Could you check a few things on this model? Use its own coordinates, in mm. A direction names the side the tool comes from. Coordinates: 2 decimals unless noted, no trailing zeros. Order: outer loops, then holes, each group sorted by start corner. A loop starts at its lowest first (then second) coordinate and runs counter-clockwise, first axis right, second up. Notation, with made-up numbers: (-7.75, -33) - (40.25, -33) arc R23 ccw to (40.25, -18) - close; hole circle Ø6 at (-7.75, 51). An arc over 180 degrees is marked (long way). Answer as a JSON object with one key per item and string values. Group by question number.
(1) Which directions (+Z, -Z, +X, -X, +Y, -Y) give clear straight access to the entire face, cutting with the end or side of a thin tool? Please do faces 1 (the flat face through (29.163, 14, 6)), 2 (the flat face through (9, 26, 1)), 3 (the flat face through (20, 58, 4)).
(2) Imagine slicing it at B-B, the plane x = 31. Write out the boundary of the cut face in (y, z), and give its area (3 significant figures).
(3) We'd pull the mould along X, two halves only. Please class faces 4 (the flat face through (20, 28, 3)), 5 (the flat face through (20, 0, 4)): pulls with the +X half, pulls with the -X half, needs draft (parallel to the pull), parting line crosses it, or undercut.
(4) Will these pins go through, and if not, where does the flat tip stop? P1, Ø1.2, axis at x = 28, y = 16, coming from the +Z side; P2, Ø0.9, axis at x = 23, y = 21.5, coming from the -Z side; P3, Ø2, axis at x = 18.5, y = 19, coming from the +Z side.
(5) Imagine slicing it at A-A, the plane y = 33. Write out the boundary of the cut face in (x, z), and give its area (3 significant figures).
(6) Please list where these lines run through material, in increasing order: probe 1 along Y at (x, z) = (5, 2); probe 2 along X at (y, z) = (18.5, 5.75); probe 3 along X at (y, z) = (46.5, 6.5).
(7) Imagine slicing it at C-C, the plane y = 4.5. Write out the boundary of the cut face in (x, z), and give its area (3 significant figures).
(8) Imagine slicing it at D-D, the plane z = 2.75. Write out the boundary of the cut face in (x, y).
from build123d import *

# Parameters (mm, degrees)
SKETCH1_W           = 60
SKETCH1_H           = 40
BOSS_EXTRUDE1_DEPTH = 8
SKETCH3_R           = 1.15
CUT_EXTRUDE2_DEPTH  = 73.553428589
SKETCH7_W           = 25
SKETCH7_H           = 30
CUT_EXTRUDE6_DEPTH  = 73.553428589
SKETCH8_W           = 18.2
SKETCH8_H           = 45
CUT_EXTRUDE7_DEPTH  = 2
SKETCH9_W           = 2.5
SKETCH9_H           = 25
CUT_EXTRUDE8_DEPTH  = 1.5
SKETCH10_W          = 18.2
SKETCH10_H          = 0.8
BOSS_EXTRUDE2_DEPTH = 1
SKETCH11_W          = 5
SKETCH11_H          = 3
SKETCH11_W_2        = 6
SKETCH11_H_2        = 11
CUT_EXTRUDE9_DEPTH  = 1.5


with BuildPart() as part:
    # Sketch1 → Boss-Extrude1 (new body)
    with BuildSketch(Plane(origin=(0, 0, 0), x_dir=(0, 1, 0), z_dir=(0, 0, 1))):
        with Locations((30, -20)):
            Rectangle(SKETCH1_W, SKETCH1_H)
    extrude(amount=BOSS_EXTRUDE1_DEPTH)

    # Sketch3 → Cut-Extrude2 (cut, through all)
    with BuildSketch(Plane.XY.offset(8)):
        with Locations((5, 4.5)):
            Circle(SKETCH3_R)
        with Locations((35, 4.5)):
            Circle(SKETCH3_R)
        with Locations((5, 55.5)):
            Circle(SKETCH3_R)
        with Locations((35, 55.5)):
            Circle(SKETCH3_R)
    extrude(amount=-CUT_EXTRUDE2_DEPTH, mode=Mode.SUBTRACT)

    # Sketch7 → Cut-Extrude6 (cut, through all)
    with BuildSketch(Plane.XY.offset(8)):
        with Locations((20, 43)):
            Rectangle(SKETCH7_W, SKETCH7_H)
    extrude(amount=-CUT_EXTRUDE6_DEPTH, mode=Mode.SUBTRACT)

    # Sketch8 → Cut-Extrude7 (cut)
    with BuildSketch(Plane.XY.offset(8)):
        with Locations((20.062509857, 22.5)):
            Rectangle(SKETCH8_W, SKETCH8_H)
    extrude(amount=-CUT_EXTRUDE7_DEPTH, mode=Mode.SUBTRACT)

    # Sketch9 → Cut-Extrude8 (cut)
    with BuildSketch(Plane.XY.offset(6)):
        with Locations((12.212509857, 15.5)):
            Rectangle(SKETCH9_W, SKETCH9_H)
        with Locations((27.912509857, 15.5)):
            Rectangle(SKETCH9_W, SKETCH9_H)
    extrude(amount=-CUT_EXTRUDE8_DEPTH, mode=Mode.SUBTRACT)

    # Sketch10 → Boss-Extrude2 (add)
    with BuildSketch(Plane.XY.offset(6)):
        with Locations((20.062509857, 0.4)):
            Rectangle(SKETCH10_W, SKETCH10_H)
    extrude(amount=BOSS_EXTRUDE2_DEPTH)

    # Sketch11 → Cut-Extrude9 (cut)
    with BuildSketch(Plane(origin=(0, 0, 0), x_dir=(1, 0, 0), z_dir=(0, 0, -1))):
        with Locations((23.5, -22.4)):
            Rectangle(SKETCH11_W, SKETCH11_H)
        with Locations((12, -28.5)):
            Rectangle(SKETCH11_W_2, SKETCH11_H_2)
    extrude(amount=-CUT_EXTRUDE9_DEPTH, mode=Mode.SUBTRACT)


solid = part.part
Result set:
{
 "1": {"face 1": "+Z", "face 2": "-Z", "face 3": "+Z, -Z"},
 "2": {"outline": "(0, 0) - (28, 0) - (28, 8) - (0, 8) - close; (58, 0) - (60, 0) - (60, 8) - (58, 8) - close", "area": "240 mm^2"},
 "3": {"face 4": "undercut", "face 5": "needs draft"},
 "4": {"P1": "stops at z = 4.5", "P2": "stops at z = 1.5", "P3": "stops at z = 6"},
 "5": {"outline": "(0, 0) - (7.5, 0) - (7.5, 8) - (0, 8) - close; (32.5, 0) - (40, 0) - (40, 8) - (32.5, 8) - close", "area": "120 mm^2"},
 "6": {"probe 1": "y = 0 to 3.35, 5.65 to 54.35, 56.65 to 60", "probe 2": "x = 0 to 10.96, 13.46 to 26.66, 29.16 to 40", "probe 3": "x = 0 to 7.5, 32.5 to 40"},
 "7": {"outline": "(0, 0) - (3.85, 0) - (3.85, 8) - (0, 8) - close; (6.15, 0) - (33.85, 0) - (33.85, 8) - (29.16, 8) - (29.16, 4.5) - (26.66, 4.5) - (26.66, 6) - (13.46, 6) - (13.46, 4.5) - (10.96, 4.5) - (10.96, 8) - (6.15, 8) - close; (36.15, 0) - (40, 0) - (40, 8) - (36.15, 8) - close", "area": "239 mm^2"},
 "8": {"outline": "(0, 0) - (40, 0) - (40, 60) - (0, 60) - close; hole circle Ø2.3 at (5, 4.5); hole circle Ø2.3 at (5, 55.5); hole (7.5, 28) - (32.5, 28) - (32.5, 58) - (7.5, 58) - close; hole circle Ø2.3 at (35, 4.5); hole circle Ø2.3 at (35, 55.5)"}
}
